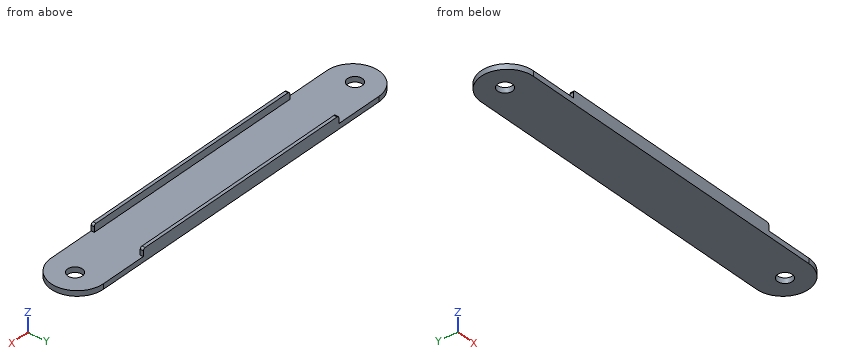
from build123d import *

# Parameters (mm, degrees)
BOSS_EXTRUDE1_DEPTH = 5
SKETCH3_W           = 220
SKETCH3_H           = 3
BOSS_EXTRUDE2_DEPTH = 7
SKETCH4_R           = 7
CUT_EXTRUDE1_DEPTH  = 7
CUT_EXTRUDE2_DEPTH  = 70


with BuildPart() as part:
    # Sketch2 → Boss-Extrude1 (new body)
    with BuildSketch(Plane.XY):
        with BuildLine():
            Line((-142.959039548, 32.18220339), (167.040960452, 32.18220339))
            ThreePointArc((167.040960452, 32.18220339), (192.040960452, 7.18220339), (167.040960452, -17.81779661))
            Line((167.040960452, -17.81779661), (-142.959039548, -17.81779661))
            ThreePointArc((-142.959039548, -17.81779661), (-167.959039548, 7.18220339), (-142.959039548, 32.18220339))
        make_face()
    extrude(amount=BOSS_EXTRUDE1_DEPTH)

    # Sketch3 → Boss-Extrude2 (add)
    with BuildSketch(Plane.XY.offset(5)):
        with Locations((12.040960452, 30.68220339)):
            Rectangle(SKETCH3_W, SKETCH3_H)
        with Locations((12.040960452, -16.31779661)):
            Rectangle(SKETCH3_W, SKETCH3_H)
    extrude(amount=BOSS_EXTRUDE2_DEPTH)

    # Sketch4 → Cut-Extrude1 (cut)
    with BuildSketch(Plane.XY.offset(5)):
        with Locations((-145.459039548, 7.18220339)):
            Circle(SKETCH4_R)
        with Locations((169.540960452, 7.18220339)):
            Circle(SKETCH4_R)
    extrude(amount=-CUT_EXTRUDE1_DEPTH, mode=Mode.SUBTRACT)

    # Sketch5 → Cut-Extrude2 (cut)
    with BuildSketch(Plane.XZ.offset(17.81779661)):
        with BuildLine():
            ThreePointArc((-97.959039548, 10), (-97.37325311, 11.414213562), (-95.959039548, 12))
            Line((-95.959039548, 12), (-97.959039548, 12))
            Line((-97.959039548, 12), (-97.959039548, 10))
        make_face()
        with BuildLine():
            Line((122.040960452, 12), (120.040960452, 12))
            ThreePointArc((120.040960452, 12), (121.455174014, 11.414213562), (122.040960452, 10))
            Line((122.040960452, 10), (122.040960452, 12))
        make_face()
    extrude(amount=-CUT_EXTRUDE2_DEPTH, mode=Mode.SUBTRACT)


solid = part.part
Read the model definition and answer for the solid it produces. Units are mm, in the model's axes. Give positions to 0.01 mm unless a question says otherwise; leave off trailing zeros. Loops run counter-clockwise (first coordinate to the right, second up) from the corner with the lowest first, then second, coordinate; pieces in that order, holes last. Notation, with made-up numbers: (1, 86) -> (51, 86) arc R25 ccw to (51, 108) -> close; hole circle Ø6 at (-0.75, 33.5). An arc over 180 degrees is marked (long way). Use a Markdown table: item, result.
Q1. Section D-D, the plane y = 23 is taken. Determine the outline of the cut face in (x, z), then the cut area to 3 significant figures.
Solved:
| item | result |
|---|---|
| outline | (-162.32, 0) -> (186.4, 0) -> (186.4, 5) -> (-162.32, 5) -> close |
| area | 1,740 mm^2 |
Q2. Section C-C, the plane y = 3.5 is taken. Determine the outline of the cut face in (x, z).
Solved:
| item | result |
|---|---|
| outline | (-167.69, 0) -> (-151.41, 0) -> (-151.41, 5) -> (-167.69, 5) -> close; (-139.51, 0) -> (163.59, 0) -> (163.59, 5) -> (-139.51, 5) -> close; (175.49, 0) -> (191.77, 0) -> (191.77, 5) -> (175.49, 5) -> close |
Q3. Find the intervals of material crossed by line 1 along Y through (x, z) = (64, 8); line 2 along X through (y, z) = (10, 3.25); line 3 along Z through (x, y) = (17.5, 21), in increasing order.
Solved:
| item | result |
|---|---|
| line 1 | y = -17.82 to -14.82, 29.18 to 32.18 |
| line 2 | x = -167.8 to -151.87, -139.05 to 163.13, 175.95 to 191.88 |
| line 3 | z = 0 to 5 |
Q4. Section B-B, the plane x = 92 is taken. Determine the outline of the cut face in (y, z).
Solved:
| item | result |
|---|---|
| outline | (-17.82, 0) -> (32.18, 0) -> (32.18, 12) -> (29.18, 12) -> (29.18, 5) -> (-14.82, 5) -> (-14.82, 12) -> (-17.82, 12) -> close |
Q5. Section A-A, the plane z = 7.5 is taken. Determine the outline of the cut face in (x, y), then the cut area to 3 significant figures.
Solved:
| item | result |
|---|---|
| outline | (-97.96, -17.82) -> (122.04, -17.82) -> (122.04, -14.82) -> (-97.96, -14.82) -> close; (-97.96, 29.18) -> (122.04, 29.18) -> (122.04, 32.18) -> (-97.96, 32.18) -> close |
| area | 1,320 mm^2 |
Q6. Each of these flat-tipped pins is pushed along its axis until it touches: pin 1 (18 mm diameter, centred on x = -145.46, y = 7.18, fed in from +Z); pin 2 (1.5 mm diameter, centred on y = -16.5, z = 7.5, fed in from -X); pin 3 (11 mm diameter, centred on x = 169.54, y = 7.18, fed in from +Z); pin 4 (5 mm diameter, centred on y = -11.5, z = 1, fed in from -X). Where does it stop, or does it pass through?
Solved:
| item | result |
|---|---|
| pin 1 | stops at z = 5 |
| pin 2 | stops at x = -97.96 |
| pin 3 | passes through |
| pin 4 | stops at x = -162.02 |
